from build123d import *

# Parameters (mm, degrees)
F0_W     = 36
F0_H     = 36
F0_R     = 1.55
F1_DEPTH = 2
F2_W     = 2.7
F2_H     = 4.2
F2_W_2   = 3.866767
F2_H_2   = 5.045659
F2_W_3   = 2.263
F2_H_3   = 0.99
F2_W_4   = 0.951673
F2_H_4   = 1.824041
F2_W_5   = 0.951672
F3_DEPTH = 1.2
F4_W     = 7.152574
F4_H     = 6.745152
F4_H_2   = 6.741168
F5_DEPTH = 2.5
F6_R     = 3


with BuildPart() as f1:
    # F0 (on Top) → F1 (new body)
    with BuildSketch(Plane.XY):
        Rectangle(F0_W, F0_H)
        with Locations((-15.25, -15.25)):
            Circle(F0_R, mode=Mode.SUBTRACT)
        with Locations((15.25, -15.25)):
            Circle(F0_R, mode=Mode.SUBTRACT)
        with Locations((-15.25, 15.25)):
            Circle(F0_R, mode=Mode.SUBTRACT)
        with Locations((15.25, 15.25)):
            Circle(F0_R, mode=Mode.SUBTRACT)
    extrude(amount=F1_DEPTH)

    # F2 (on face) → F3 (join)
    with BuildSketch(Plane.XY.offset(2)):
        with Locations((-9.406283, 9.322272)):
            Rectangle(F2_W, F2_H)
        with Locations((-9.406283, -4.017373)):
            Rectangle(F2_W, F2_H)
        with Locations((-5.734202, 9.322272)):
            Rectangle(F2_W, F2_H)
        with Locations((-5.734202, -4.017373)):
            Rectangle(F2_W, F2_H)
        with Locations((-2.062121, 9.322272)):
            Rectangle(F2_W, F2_H)
        with Locations((-2.062121, -4.017373)):
            Rectangle(F2_W, F2_H)
        with Locations((3.909136, 7.057227)):
            Rectangle(F2_W_2, F2_H_2)
        with Locations((4.035184, -6.228325)):
            Rectangle(F2_W_2, F2_H_2)
        with Locations((9.751364, 9.226358)):
            Rectangle(F2_W_3, F2_H_3)
        with Locations((9.751364, 7.733123)):
            Rectangle(F2_W_3, F2_H_3)
        with Locations((9.751364, 6.239888)):
            Rectangle(F2_W_3, F2_H_3)
        with Locations((9.751364, 4.746653)):
            Rectangle(F2_W_3, F2_H_3)
        with Locations((9.751364, 3.253418)):
            Rectangle(F2_W_3, F2_H_3)
        with Locations((9.994023, -4.120474)):
            Rectangle(F2_W_3, F2_H_3)
        with Locations((9.994023, -5.613709)):
            Rectangle(F2_W_3, F2_H_3)
        with Locations((9.994023, -7.106944)):
            Rectangle(F2_W_3, F2_H_3)
        with Locations((9.994023, -8.600179)):
            Rectangle(F2_W_3, F2_H_3)
        with Locations((9.994023, -10.093414)):
            Rectangle(F2_W_3, F2_H_3)
        with Locations((0.984356, 3.291811)):
            Rectangle(F2_W_3, F2_H_3)
        with Locations((6.319413, 3.225123)):
            Rectangle(F2_W_3, F2_H_3)
        with Locations((1.351141, -10.045832)):
            Rectangle(F2_W_3, F2_H_3)
        with Locations((6.750784, -10.012488)):
            Rectangle(F2_W_3, F2_H_3)
        with Locations((-10.585669, -16.109239)):
            Rectangle(F2_W_4, F2_H_4)
        with Locations((-9.228029, -16.109239)):
            Rectangle(F2_W_4, F2_H_4)
        with Locations((2.207651, -16.109239)):
            Rectangle(F2_W_4, F2_H_4)
        with Locations((3.96747, -16.109239)):
            Rectangle(F2_W_5, F2_H_4)
    extrude(amount=F3_DEPTH)

    # F4 (on face) → F5 (join)
    with BuildSketch(Plane.XY.offset(2)):
        with Locations((-5.296527, 2.516344)):
            Rectangle(F4_W, F4_H)
        with Locations((-5.296527, -10.817411)):
            Rectangle(F4_W, F4_H_2)
    extrude(amount=F5_DEPTH)

    # F6
    f6_edges = [f1.edges().sort_by_distance(p)[0] for p in [
        (-18, 18, 1),
        (-18, -18, 1),
        (18, -18, 1),
        (18, 18, 1),
    ]]
    fillet(f6_edges, radius=F6_R)


solid = f1.part
CAD build for the part. Positions are in the model's coordinates, mm. A direction names the side the tool comes from. Give positions to 0.01 mm unless a question says otherwise; leave off trailing zeros. Write each loop counter-clockwise with the first axis right and the second up, starting at its lowest first coordinate (ties: lowest second). Pieces come first, ordered by that corner, then holes. Notation, with made-up numbers: M -40,50.5 L 9,50.5 A13 ccw 9,55.5 Z; hole C 57,17.5 d1. An arc over 180 degrees is marked long. Put each result on its own line as item: value. Start each with the question number.
(1) Band-saw the part on C-C, the plane z = 3.9. Write the cut outline in (x, y).
(2) Which spindle directions (+Z, -Z, +X, -X, +Y, -Y) get a long thin tool onto all of the face, cutting with end or side? Do faces 1 (the face through (2.683, -16, 3)), 2 (the face through (-5, 5.889, 3)), 3 (the face through (10, 5.242, 3)). Say none if no direction does.
(3) Flat gauge pins, fed straight in: pin 1 Ø0.6 at (y, z) = (-16, 3) entering from -X; pin 2 Ø1.3 at (x, y) = (-9.5, -3) entering from +Z; pin 3 Ø1.3 at (x, z) = (9.5, 3) entering from -Y. Where does each tip first touch, or does it go through?
(4) Band-saw the part on B-B, the plane y = -12. Write the cut outline in (x, z).
(5) Mould opens along X. For faces 4 (the face through (8.62, 8, 3)), 5 (the face through (-0.147, 3, 3)), 6 (the face through (-2, -6.117, 3)), 7 (the face through (-17.14, -17.1, 1.01)) say: +X half, -X half, draft (parallel to the pull), parting line (faces both ways), or undercut.
(6) Band-saw the part on D-D, the plane x = 4. Write the cut outline in (y, z), and give its area (3 significant figures).
(7) Band-saw the part on A-A, the plane z = 0.6. Write the cut outline in (x, y), and give its area (3 significant figures).
(8) Probe L1, parallel to Y at x = 15.25, z = 0.7; L2, parallel to X at y = 15, z = 0.2; L3, parallel to Z at x = 1.5, y = -5.5. List the from-to ranges inside material, lowest first.
Response values:
1. outline: M -8.87,-14.19 L -1.72,-14.19 L -1.72,-7.45 L -8.87,-7.45 Z; M -8.87,-0.86 L -1.72,-0.86 L -1.72,5.89 L -8.87,5.89 Z
2. face 1: +Z, -Y
2. face 2: +Z, -X
2. face 3: +Z, +X
3. pin 1: stops at x = -11.06
3. pin 2: stops at z = 3.2
3. pin 3: stops at y = -10.59
4. outline: M -18,0 L 18,0 L 18,2 L -1.72,2 L -1.72,4.5 L -8.87,4.5 L -8.87,2 L -18,2 Z
5. face 4: undercut
5. face 5: undercut
5. face 6: draft
5. face 7: -X half
6. outline: M -18,0 L 18,0 L 18,2 L 9.58,2 L 9.58,3.2 L 4.53,3.2 L 4.53,2 L -3.71,2 L -3.71,3.2 L -8.75,3.2 L -8.75,2 L -15.2,2 L -15.2,3.2 L -17.02,3.2 L -17.02,2 L -18,2 Z
6. area: 86.3 mm2
7. outline: M -18,-15 A3 ccw -15,-18 L 15,-18 A3 ccw 18,-15 L 18,15 A3 ccw 15,18 L -15,18 A3 ccw -18,15 Z; hole C -15.25,-15.25 d3.1; hole C -15.25,15.25 d3.1; hole C 15.25,-15.25 d3.1; hole C 15.25,15.25 d3.1
7. area: 1,260 mm2
8. L1: y = -17.99 to -16.8, -13.7 to 13.7, 16.8 to 17.99
8. L2: x = -18 to -16.78, -13.72 to 13.72, 16.78 to 18
8. L3: z = 0 to 2
